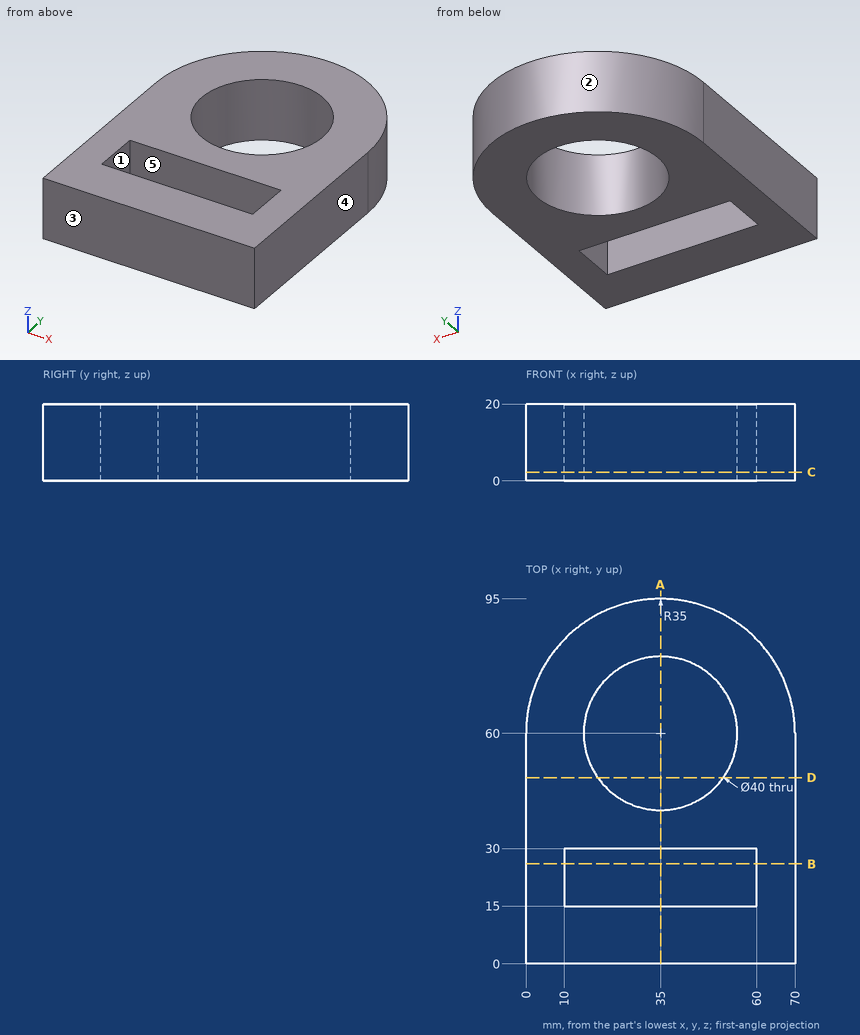
Input: dimensioned drawing with shaded views. Units: mm. Origin: part minimum x, y, z. A direction names the side the tool comes from. Give positions to 0.01 mm unless a question says otherwise; leave off trailing zeros. Write each loop counter-clockwise with the first axis right and the second up, starting at its lowest first coordinate (ties: lowest second). Pieces come first, ordered by that corner, then holes. Notation, with made-up numbers: M 3,62.5 L 27,62.5 A7 cw 27,70.5 Z; hole C 77.5,31 d10. An arc over 180 degrees is marked long. Return JSON: item names as keys, results as strings. Group by question number.
1) Set-up query: the marked faces 1 and 2. Return all of +Z, -Z, +X, -X, +Y, -Y with unobstructed straight access to the full face (end or side cutting, diameter ignored); none if empty.
2) Cut plane B-B, the plane y = 26. Output: boundary loops of the cut face in (x, z).
3) Cut plane A-A, the plane x = 35. Output: boundary loops of the cut face in (y, z).
4) Pin query (flat end, axial travel): P1, Ø6, axis at y = 83.5, z = 15, coming from the +X side; P2, Ø6, axis at x = 39.5, z = 10, coming from the +Y side; P3, Ø1.5, axis at y = 78.5, z = 9, coming from the +X side. Return the tip coordinate at first contact, or that it passes through.
5) Cut plane D-D, the plane y = 48.5. Output: boundary loops of the cut face in (x, z), plus the area to 3 significant figures.
6) Cut plane C-C, the plane z = 2.25. Output: boundary loops of the cut face in (x, y), plus the area to 3 significant figures.
7) Material intervals for line 1 along Y through (x, z) = (35, 16.25); line 2 along Y through (x, z) = (44, 8.5); line 3 along X through (y, z) = (16, 4), sorted ascending. Write a range as [from, to].
8) Pull-direction query (Y, two-part tool) for the marked faces 3, 4 and 5; classes: pulls with the +Y half, pulls with the -Y half, needs draft (parallel to the pull), parting line crosses it, or undercut.
Recorded:
{
 "1": {"face 1": "+Z, -Z", "face 2": "+Z, -Z, +Y"},
 "2": {"outline": "M 0,0 L 10,0 L 10,20 L 0,20 Z; M 60,0 L 70,0 L 70,20 L 60,20 Z"},
 "3": {"outline": "M 0,0 L 15,0 L 15,20 L 0,20 Z; M 30,0 L 40,0 L 40,20 L 30,20 Z; M 80,0 L 95,0 L 95,20 L 80,20 Z"},
 "4": {"P1": "stops at x = 63.37", "P2": "stops at y = 94.97", "P3": "stops at x = 65.17"},
 "5": {"outline": "M 0,0 L 18.64,0 L 18.64,20 L 0,20 Z; M 51.36,0 L 70,0 L 70,20 L 51.36,20 Z", "area": "745 mm²"},
 "6": {"outline": "M 0,0 L 70,0 L 70,60 A35 ccw 0,60 Z; hole M 10,15 L 60,15 L 60,30 L 10,30 Z; hole C 35,60 d40", "area": "4,120 mm²"},
 "7": {"line 1": "y = [0, 15], [30, 40], [80, 95]", "line 2": "y = [0, 15], [30, 42.14], [77.86, 93.82]", "line 3": "x = [0, 10], [60, 70]"},
 "8": {"face 3": "pulls with the -Y half", "face 4": "needs draft", "face 5": "undercut"}
}
